Can you work these out from the model? Positions are in its coordinate system, mm. Face numbers are marked on the shaded views. Give positions to 0.01 mm unless a question says otherwise; leave off trailing zeros. Write each loop counter-clockwise with the first axis right and the second up, starting at its lowest first coordinate (ties: lowest second). Pieces come first, ordered by that corner, then holes.
1. I'm going to push flat-ended pins straight in: pin 1 (3 mm diameter, centred on y = -629, z = 89.5, fed in from +X); pin 2 (10 mm diameter, centred on y = -352.5, z = 37, fed in from +X); pin 3 (6 mm diameter, centred on x = 35, z = 28.5, fed in from -Y). Where does each tip first touch, or does it pass through?
2. Suppose I cut it at D-D (y = -512). Please give me the cut outline in (x, z), and give its area (3 significant figures).
3. Thinking about a two-plate mould opening in Y: for the marked faces 1, 2, 3 and 4, which applies, pulls with the +Y half, pulls with the -Y half, needs draft (parallel to the pull), parting line crosses it, or undercut?
4. Suppose I cut it at A-A (x = 0). Please give me the cut outline in (y, z), and give its area (3 significant figures).
5. Suppose I cut it at C-C (y = -125). Please give me the cut outline in (x, z), and give its area (3 significant figures).
6. Suppose I cut it at B-B (z = 0). Please give me the cut outline in (x, y).
7. If I drill on probe 1 along Y at (x, z) = (113, 81.5); probe 2 along X at (y, z) = (-709.5, 187); probe 3 along X at (y, z) = (-590.5, 11), over which ranges is the centre line in solid material (lowest first)?
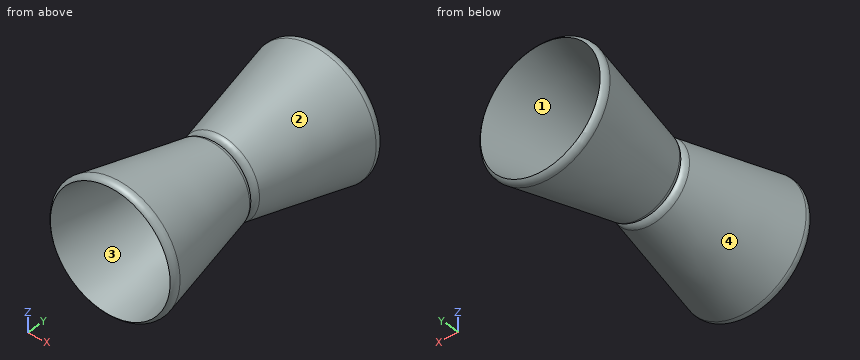
```python
from build123d import *

# Parameters (mm, degrees)
FILLET1_R = 30


# Read off the part's stored shape, not the designer's step: Mirror1
with BuildPart() as part:
    # Sketch1 → Revolve1 (revolve)
    with BuildSketch(Plane.XY, mode=Mode.PRIVATE) as revolve1_sk:
        Polygon((0, -330.841690926), (0, -380.841690926), (160, -380.841690926), (270.482436132, 119.158309074), (250, 119.158309074), (150.565807481, -330.841690926), align=None)
    revolve(revolve1_sk.sketch.rotate(Axis((0, -330.841690926, 0), (0, -1, 0)), 180), axis=Axis((0, -330.841690926, 0), (0, -1, 0)))

    # Fillet1
    # the kernel refuses this fillet: 30 mm, written as the material it takes off along each edge
    with BuildSketch(Plane(origin=(0, -380.841690926, 0), x_dir=(-1, 0, 0), z_dir=(0, 0, 1))) as fillet1_piece_1:
        with BuildLine():
            CenterArc((160 - FILLET1_R * 0.803156934346, -FILLET1_R), FILLET1_R, 12.46013877, 77.53986123)
            Line((160 + FILLET1_R * 0.173289415634, -FILLET1_R * 0.784239657004), (160 + FILLET1_R * 0.192818342634, -FILLET1_R * 0.779924450144))
            Line((160 + FILLET1_R * 0.192818342634, -FILLET1_R * 0.779924450144), (160 + FILLET1_R * 0.0160631386869, FILLET1_R * 0.02))
            Line((160 + FILLET1_R * 0.0160631386869, FILLET1_R * 0.02), (160 - FILLET1_R * 0.803156934346, FILLET1_R * 0.02))
            Line((160 - FILLET1_R * 0.803156934346, FILLET1_R * 0.02), (160 - FILLET1_R * 0.803156934346, 0))
        make_face()
    revolve(axis=Axis((0, -380.841690926, 0), (0, -1, 0)), mode=Mode.SUBTRACT)
    with BuildSketch(Plane(origin=(0, 119.158309074, 0), x_dir=(-1, 0, 0), z_dir=(0, 0, 1))) as fillet1_piece_2:
        with BuildLine():
            CenterArc((234.132912434, 25.460469991), FILLET1_R, 301.931359404, 70.528779366)
            Line((250, 0), (250.317341751, -0.5092094))
            ThreePointArc((250.317341751, -0.5092094), (260.241218066, -0.6), (270.482436132, -0.6))
            Line((270.482436132, -0.6), (271.068303942, 0.129456206))
            Line((271.068303942, 0.129456206), (264.012170744, 32.062736487))
            Line((264.012170744, 32.062736487), (263.426302934, 31.933280281))
        make_face()
    revolve(axis=Axis((0, 119.158309074, 0), (0, -1, 0)), mode=Mode.SUBTRACT)

    # Mirror1 outline → Mirror1 (revolve)
    with BuildSketch(Plane.XY):
        with BuildLine():
            Line((0, -380.841690926), (0, -430.841690926))
            Line((0, -430.841690926), (150.565807481, -430.841690926))
            Line((150.565807481, -430.841690926), (250, -880.841690926))
            ThreePointArc((250, -880.841690926), (261.787944384, -867.008740354), (263.426302934, -848.908410644))
            Line((263.426302934, -848.908410644), (165.198682469, -404.368880636))
            ThreePointArc((165.198682469, -404.368880636), (154.691133597, -387.451689764), (135.90529197, -380.841690926))
            Line((135.90529197, -380.841690926), (0, -380.841690926))
        make_face()
    revolve(axis=Axis((0, 0, 0), (0, 1, 0)))


solid = part.part
```
Checks:
1. pin 1: stops at x = 196.08
1. pin 2: stops at x = 163.66
1. pin 3: stops at y = -430.84
2. outline: circle Ø377.96 at (0, 0); hole circle Ø337 at (0, 0)
2. area: 23,000 mm2
3. face 1: pulls with the +Y half
3. face 2: undercut
3. face 3: pulls with the -Y half
3. face 4: undercut
4. outline: (-880.84, -250) arc R30 ccw to (-848.91, -263.43) - (-404.37, -165.2) arc R30 ccw to (-380.84, -135.91) arc R30 ccw to (-357.31, -165.2) - (87.23, -263.43) arc R30 ccw to (119.16, -250) - (-330.84, -150.57) - (-330.84, 150.57) - (119.16, 250) arc R30 ccw to (87.23, 263.43) - (-357.31, 165.2) arc R30 ccw to (-380.84, 135.91) arc R30 ccw to (-404.37, 165.2) - (-848.91, 263.43) arc R30 ccw to (-880.84, 250) - (-430.84, 150.57) - (-430.84, -150.57) - close
4. area: 68,700 mm2
5. outline: circle Ø433.06 at (0, 0); hole circle Ø392.1 at (0, 0)
5. area: 26,500 mm2
6. outline: (-263.43, -848.91) arc R30 ccw to (-250, -880.84) - (-150.57, -430.84) - (150.57, -430.84) - (250, -880.84) arc R30 ccw to (263.43, -848.91) - (165.2, -404.37) arc R30 ccw to (135.91, -380.84) arc R30 ccw to (165.2, -357.31) - (263.43, 87.23) arc R30 ccw to (250, 119.16) - (150.57, -330.84) - (-150.57, -330.84) - (-250, 119.16) arc R30 ccw to (-263.43, 87.23) - (-165.2, -357.31) arc R30 ccw to (-135.91, -380.84) arc R30 ccw to (-165.2, -404.37) - close
7. probe 1: y = -430.84 to -381.04, -380.65 to -330.84
7. probe 2: x = -138.36 to -100.17, 100.17 to 138.36
7. probe 3: x = -206.03 to -185.52, 185.52 to 206.03
